Part print with two shaded views. Sizes in mm from the minimum x, y, z corner. A direction names the side the tool comes from. Round coordinates to 2 decimals unless told otherwise and drop trailing zeros. Write each loop counter-clockwise with the first axis right and the second up, starting at its lowest first coordinate (ties: lowest second). Pieces come first, ordered by that corner, then holes. Notation, with made-up numbers: M 60.5,76 L 88.5,76 A14 ccw 88.5,83 Z; hole C 39,-16 d5. An arc over 180 degrees is marked long. One line per question, with ' | ' between items. Start each with the question number.
1) Saw through at D-D (x = 6). List the corners of the cut face in (y, z), plus the area to 3 significant figures.
2) Drop flat-ended pins along their axis: pin 1 Ø5 at (x, y) = (3.5, 19.5) entering from +Z; pin 2 Ø1 at (y, z) = (13, 20.5) entering from +X; pin 3 Ø1.5 at (y, z) = (13, 20) entering from +X. Give the stop position or say it passes through.
3) Saw through at C-C (z = 15.5). List the corners of the cut face in (x, y).
4) Wall check: probe 1 along Y at (x, z) = (11, 5.75); probe 2 along Z at (x, y) = (16.75, 5); probe 3 along Z at (x, y) = (16.5, 19). Give the ranges that are in metal, low to high. Write a range as [from, to].
5) Saw through at A-A (x = 11). List the corners of the cut face in (y, z), plus the area to 3 significant figures.
6) Mould opens along X. For the marked faces 4, 5, 6 and 7 say: pulls with the +X half, pulls with the -X half, needs draft (parallel to the pull), parting line crosses it, or undercut.
7) Tool access for the marked faces 1, 2 and 3: list every direction of +Z, -Z, +X, -X, +Y, -Y with a clear straight run to the whole face (end or side of a thin tool).
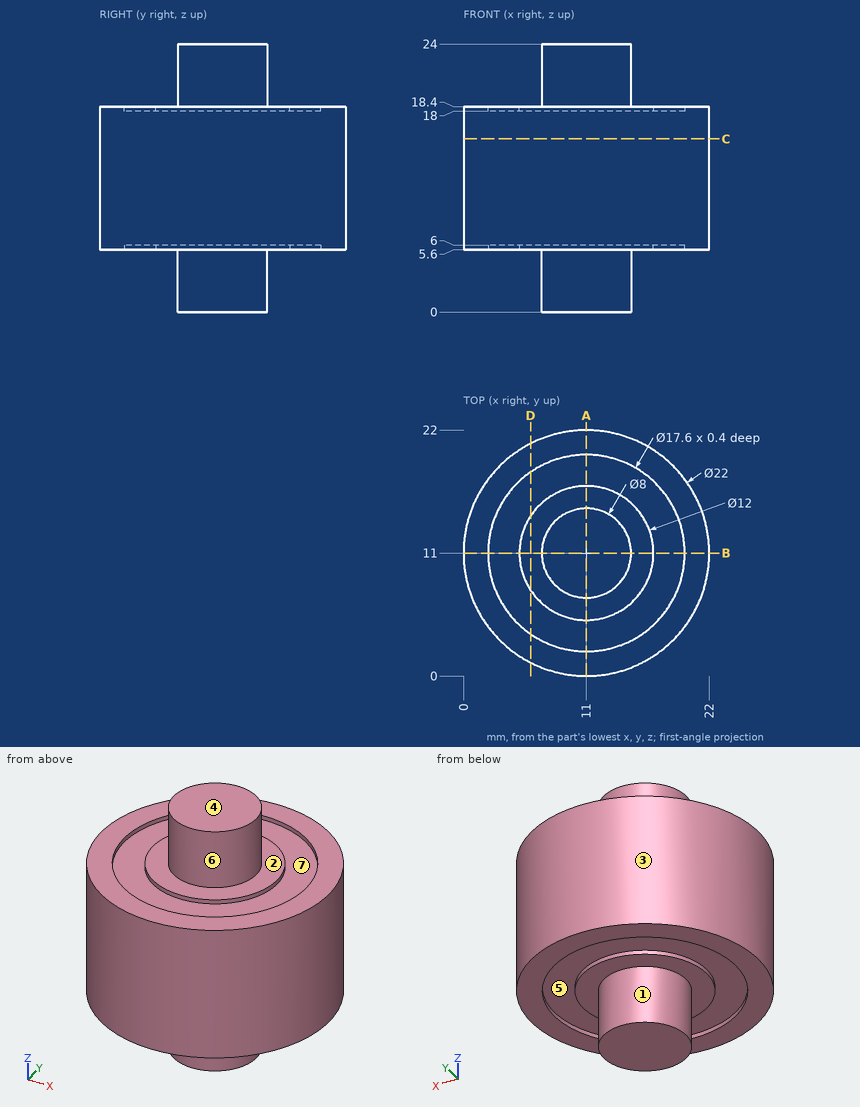
Answer key:
1) outline: M 1.2,5.6 L 3.76,5.6 L 3.76,6 L 7.68,6 L 7.68,5.6 L 14.32,5.6 L 14.32,6 L 18.24,6 L 18.24,5.6 L 20.8,5.6 L 20.8,18.4 L 18.24,18.4 L 18.24,18 L 14.32,18 L 14.32,18.4 L 7.68,18.4 L 7.68,18 L 3.76,18 L 3.76,18.4 L 1.2,18.4 Z | area: 245 mm2
2) pin 1: stops at z = 18.4 | pin 2: stops at x = 14.71 | pin 3: stops at x = 14.8
3) outline: C 11,11 d22
4) probe 1: y = [0, 2.2], [5, 17], [19.8, 22] | probe 2: z = [6, 18] | probe 3: z = [5.6, 18.4]
5) outline: M 0,5.6 L 2.2,5.6 L 2.2,6 L 5,6 L 5,5.6 L 7,5.6 L 7,0 L 15,0 L 15,5.6 L 17,5.6 L 17,6 L 19.8,6 L 19.8,5.6 L 22,5.6 L 22,18.4 L 19.8,18.4 L 19.8,18 L 17,18 L 17,18.4 L 15,18.4 L 15,24 L 7,24 L 7,18.4 L 5,18.4 L 5,18 L 2.2,18 L 2.2,18.4 L 0,18.4 Z | area: 367 mm2
6) face 4: needs draft | face 5: undercut | face 6: parting line crosses it | face 7: undercut
7) face 1: -Z | face 2: +Z | face 3: +Z, -Z
